from build123d import *

# Parameters (mm, degrees)
BOSS_EXTRUDE1_DEPTH     = 215.9
CUT_EXTRUDE1_DEPTH      = 235.52055347
CUT_EXTRUDE1_DEPTH_BACK = 235.52055347
CUT_EXTRUDE2_DEPTH      = 235.52055347
CUT_EXTRUDE2_DEPTH_BACK = 235.52055347
CUT_EXTRUDE3_DEPTH      = 267.567675507
CUT_EXTRUDE3_DEPTH_BACK = 267.567675507


with BuildPart() as part:
    # Sketch1 → Boss-Extrude1 (new, symmetric)
    with BuildSketch(Plane.XY):
        with BuildLine():
            Line((-63.5, -50.8), (63.5, -50.8))
            ThreePointArc((63.5, -50.8), (72.480256121, -47.080256121), (76.2, -38.1))
            Line((76.2, -38.1), (76.2, 38.1))
            ThreePointArc((76.2, 38.1), (72.480256121, 47.080256121), (63.5, 50.8))
            Line((63.5, 50.8), (-63.5, 50.8))
            ThreePointArc((-63.5, 50.8), (-72.480256121, 47.080256121), (-76.2, 38.1))
            Line((-76.2, 38.1), (-76.2, -38.1))
            ThreePointArc((-76.2, -38.1), (-72.480256121, -47.080256121), (-63.5, -50.8))
        make_face()
        with BuildLine():
            Line((-63.5, 44.45), (63.5, 44.45))
            ThreePointArc((63.5, 44.45), (67.990128061, 42.590128061), (69.85, 38.1))
            Line((69.85, 38.1), (69.85, -38.1))
            ThreePointArc((69.85, -38.1), (67.990128061, -42.590128061), (63.5, -44.45))
            Line((63.5, -44.45), (-63.5, -44.45))
            ThreePointArc((-63.5, -44.45), (-67.990128061, -42.590128061), (-69.85, -38.1))
            Line((-69.85, -38.1), (-69.85, 38.1))
            ThreePointArc((-69.85, 38.1), (-67.990128061, 42.590128061), (-63.5, 44.45))
        make_face(mode=Mode.SUBTRACT)
    extrude(amount=BOSS_EXTRUDE1_DEPTH, both=True)

    # Sketch2 → Cut-Extrude1 (cut, two sides: drawn at the far end of the back side and taken through both)
    with BuildSketch(Plane(origin=(0, 0, 0), x_dir=(0, 0, -1), z_dir=(1, 0, 0)).offset(-CUT_EXTRUDE1_DEPTH_BACK)):
        Polygon((-215.9, 50.8), (-215.9, -50.8), (-159.369185588, -50.8), (-159.369185588, -38.1), (-212.725, 38.1), (-212.725, 50.8), align=None)
    extrude(amount=CUT_EXTRUDE1_DEPTH + CUT_EXTRUDE1_DEPTH_BACK, mode=Mode.SUBTRACT)

    # Sketch3 → Cut-Extrude2 (cut, two sides: drawn at the far end of the back side and taken through both)
    with BuildSketch(Plane(origin=(0, 0, 0), x_dir=(0, 0, -1), z_dir=(1, 0, 0)).offset(-CUT_EXTRUDE2_DEPTH_BACK)):
        Polygon((70.328712905, 76.692890201), (278.875695835, 76.692890201), (278.875695835, -66.353510659), (183.855194167, -85.439727725), align=None)
    extrude(amount=CUT_EXTRUDE2_DEPTH + CUT_EXTRUDE2_DEPTH_BACK, mode=Mode.SUBTRACT)

    # Sketch4 → Cut-Extrude3 (cut, two sides: drawn at the far end of the back side and taken through both)
    with BuildSketch(Plane(origin=(76.2, 0, 0), x_dir=(0, 0, -1), z_dir=(1, 0, 0)).offset(-CUT_EXTRUDE3_DEPTH_BACK)):
        Polygon((51.667098459, -105.135311235), (172.443519022, -20.566751119), (188.243794301, -73.434684409), align=None)
    extrude(amount=CUT_EXTRUDE3_DEPTH + CUT_EXTRUDE3_DEPTH_BACK, mode=Mode.SUBTRACT)


solid = part.part
Read the model definition and answer for the solid it produces. Units are mm, in the model's axes. A direction names the side the tool comes from. Give positions to 0.01 mm unless a question says otherwise; leave off trailing zeros. Write each loop counter-clockwise with the first axis right and the second up, starting at its lowest first coordinate (ties: lowest second). Pieces come first, ordered by that corner, then holes. Notation, with made-up numbers: (12.25, -26.75) - (33.25, -26.75) arc R14 ccw to (33.25, 0.25) - close; hole circle Ø8 at (50.5, -20.5). An arc over 180 degrees is marked (long way). Use CSV: the item, a comma, the result in double quotes. Start each with the question number.
Item 1: The part is cut by section C-C, the plane y = 26. Give the vertices of the cut face in (x, z), and give its area (3 significant figures).
Item 2: Consider line 1 (X direction, y = 28.5, z = -29); line 2 (Y direction, x = -14.5, z = 123.5); line 3 (Y direction, x = 57, z = 182). Determine where each line is inside the solid, lowest interval first.
Item 3: A flat-ended cylindrical pin translates along its axis: P1, Ø4, axis at x = 35, y = -43, coming from the +Z side. Find the tip coordinate at first contact, or state that the pin passes through.
Item 4: The part is cut by section D-D, the plane z = -114.5. Give the vertices of the cut face in (x, y), and give its area (3 significant figures).
Item 5: The part is cut by section B-B, the plane z = 98.5. Give the vertices of the cut face in (x, y).
Item 6: The mould has two halves that part along Y. Classify faces 4 (the cylindrical face through (67.94, 42.64, 59.86)), 5 (the cylindrical face through (72.38, -47.18, 8.13)), 6 (the flat face through (-1, 47, 212.725)): pulls with the +Y half, pulls with the -Y half, needs draft (parallel to the pull), parting line crosses it, or undercut.
Item 7: For faces 1 (the cylindrical face through (-67.94, -42.64, 8.13)), 2 (the flat face through (-1, -47, 159.369)), 3 (the cylindrical face through (-72.58, -46.98, 8.13)), determine the directions among +Z, -Z, +X, -X, +Y, -Y from which every point of the face is accessible in a straight line to the end or side of a thin tool.
Item 8: The part is cut by section A-A, the plane x = 25. Give the vertices of the cut face in (y, z) (3 decimals).
Taken from the geometry:
1,outline,"(-76.2, -105.82) - (-69.85, -105.82) - (-69.85, 204.25) - (-76.2, 204.25) - close; (69.85, -105.82) - (76.2, -105.82) - (76.2, 204.25) - (69.85, 204.25) - close"
1,area,"3,940 mm2"
2,line 1,"-76.2 to -69.85, 69.85 to 76.2"
2,line 2,"-50.8 to -44.45, 44.45 to 50.8"
2,line 3,"44.45 to 50.8"
3,P1,"z = 159.37"
4,outline,"(-76.2, -38.1) arc R12.7 ccw to (-63.5, -50.8) - (63.5, -50.8) arc R12.7 ccw to (76.2, -38.1) - (76.2, 13.61) - (69.85, 13.61) - (69.85, -38.1) arc R6.35 cw to (63.5, -44.45) - (-63.5, -44.45) arc R6.35 cw to (-69.85, -38.1) - (-69.85, 13.61) - (-76.2, 13.61) - close"
4,area,"1,650 mm2"
5,outline,"(-76.2, -38.1) arc R12.7 ccw to (-63.5, -50.8) - (63.5, -50.8) arc R12.7 ccw to (76.2, -38.1) - (76.2, 38.1) arc R12.7 ccw to (63.5, 50.8) - (-63.5, 50.8) arc R12.7 ccw to (-76.2, 38.1) - close; hole (-69.85, -38.1) arc R6.35 ccw to (-63.5, -44.45) - (63.5, -44.45) arc R6.35 ccw to (69.85, -38.1) - (69.85, 38.1) arc R6.35 ccw to (63.5, 44.45) - (-63.5, 44.45) arc R6.35 ccw to (-69.85, 38.1) - close"
6,face 4,"undercut"
6,face 5,"pulls with the -Y half"
6,face 6,"needs draft"
7,face 1,"+Z, -Z"
7,face 2,"+Z, +X, -X, -Y"
7,face 3,"+Z, -Z, -X, -Y"
8,outline,"(-50.8, -129.266) - (-44.45, -138.335) - (-44.45, 159.369) - (-50.8, 159.369) - close; (44.45, -92.905) - (50.8, -88.459) - (50.8, 212.725) - (44.45, 212.725) - close"
